```python
from build123d import *

# Parameters (mm, degrees)
CUT_EXTRUDE1_DEPTH = 0.5


with BuildPart() as part:
    # Sketch1 → Revolve1 (revolve)
    with BuildSketch(Plane.XY):
        with BuildLine():
            Line((0, 1.61), (1.34, 1.61))
            ThreePointArc((1.34, 1.61), (2.337020561, 1.197020561), (2.75, 0.2))
            Line((2.75, 0.2), (2.75, 0))
            Line((2.75, 0), (1.5, 0))
            Line((1.5, 0), (1.5, -6))
            Line((1.5, -6), (0, -6))
            Line((0, -6), (0, 1.61))
        make_face()
    revolve(axis=Axis((0, 9.083769969, 0), (0, -1, 0)))

    # Sketch2 → Cut-Extrude1 (cut)
    with BuildSketch(Plane(origin=(0, 1.61, 0), x_dir=(1, 0, 0), z_dir=(0, 1, 0))):
        Polygon((0.62654248, 1.085203409), (-0.62654248, 1.085203409), (-1.253084961, 0), (-0.62654248, -1.085203409), (0.62654248, -1.085203409), (1.253084961, 0), align=None)
    extrude(amount=-CUT_EXTRUDE1_DEPTH, mode=Mode.SUBTRACT)


solid = part.part
```
For this review, take the finished solid that the model builds, in its own axes (mm). Give positions to 0.01 mm unless a question says otherwise; leave off trailing zeros. Order: outer loops, then holes, each group sorted by start corner. A loop starts at its lowest first (then second) coordinate and runs counter-clockwise, first axis right, second up.
1) Wall thickness on line 1 (Z direction, x = -1.15, y = 1.25); line 2 (X direction, y = -1.5, z = -0.05); line 3 (Y direction, x = 1.1, z = 0.1): over which ranges is each line inside the solid? List them lowest first.
2) Take a section at A-A (y = -5.5). Give the boundary of the cut face in (x, z).
3) The part is to be moulded in two halves that separate along Z. For faces 1 (the face through (-1.5, -3.04, 0.07)), 2 (the face through (0, 1.11, 0)), 3 (the face through (0, -6, 0)), say which applies: released by +Z, released by -Z, zero draft, split by the parting line, or undercut.
4) Insertion check: pin 1 (1.5 mm diameter, centred on x = -1.5, y = 0, fed in from +Z); pin 2 (0.7 mm diameter, centred on x = -0.5, z = 0, fed in from +Y); pin 3 (0.6 mm diameter, centred on x = 0, y = 1.5, fed in from -Z). Each pin has a flat end and moves straight along its axis. Give the tip position at first contact, or say it passes through.
Derived:
1. line 1: z = -1.97 to -0.18, 0.18 to 1.97
1. line 2: x = -1.5 to 1.5
1. line 3: y = -6 to 1.11
2. outline: circle Ø3 at (0, 0)
3. face 1: split by the parting line
3. face 2: undercut
3. face 3: zero draft
4. pin 1: stops at z = 2.65
4. pin 2: stops at y = 1.11
4. pin 3: stops at z = -2.33
